Check sheet for the modelled part. Datum: model origin and axes. Units: mm. A direction names the side the tool comes from. Give positions to 0.01 mm unless a question says otherwise; leave off trailing zeros. Order: outer loops, then holes, each group sorted by start corner. A loop starts at its lowest first (then second) coordinate and runs counter-clockwise, first axis right, second up.
from build123d import *

# Parameters (mm, degrees)
F0_R     = 13.786
F0_R_2   = 11.5
F1_DEPTH = 107.95
F2_R     = 13.786
F2_R_2   = 11.5
F3_DEPTH = 31.75
F3_TAPER = 50
F4_T     = 2.54
F5_COUNT = 4
F6_R     = 2.54
F6_2_R   = 2.54
F6_3_R   = 2.54
F6_4_R   = 2.54


# Not quite as in the source:
# - a shell that OpenCascade refuses in one call is made with other operations: the cavity is built on its own and cut out
# - a feature names something its author has since deleted; it is built from what else it names


with BuildPart() as f1:
    # F0 (on Top) → F1 (new body)
    with BuildSketch(Plane.XY):
        Circle(F0_R)
        Circle(F0_R_2, mode=Mode.SUBTRACT)
    extrude(amount=F1_DEPTH)

    # F2 (on face) → F3 (join)
    with BuildSketch(Plane.XY.offset(107.95)):
        Circle(F2_R)
        Circle(F2_R_2, mode=Mode.SUBTRACT)
        Circle(F2_R_2)
    extrude(amount=F3_DEPTH, taper=F3_TAPER)

    # F4: shell of thickness 2.54, made by hand


with BuildPart() as f4_core1:
    # F4_t2: copy of F1
    add(f1.part)

    # the walls: a layer under each face that stays
    f4_faces = [f4_core1.faces().sort_by_distance(p)[0] for p in [
        (-13.786, 0, 53.975),
        (-9.1906666667, -9.1906666667, 0),
        (-6.893, 0, 113.7339137577),
        (-11.5, 0, 53.975),
    ]]
    thicken(f4_faces, amount=-F4_T, mode=Mode.SUBTRACT)


with BuildPart() as f1_1:
    add(f1.part)

    # what is left inside the walls is the cavity
    f4_cavity = [f4_core1.part.solids().sort_by_distance(p)[0] for p in [
        (-6.539981, 0, 110.68124),
    ]]
    add(f4_cavity, mode=Mode.SUBTRACT)


with BuildPart() as f5_1:
    # F5: instance of F1
    add(f1_1.part.rotate(Axis((0, 0, 0), (0, 0, 1)), 1 * 360 / F5_COUNT))

    # F6#2
    f6_2_edges = [f5_1.edges().sort_by_distance(p)[0] for p in [
        (0, -13.786, 107.95),
    ]]
    fillet(f6_2_edges, radius=F6_2_R)


with BuildPart() as f5_2:
    # F5: instance of F1
    add(f1_1.part.rotate(Axis((0, 0, 0), (0, 0, 1)), 2 * 360 / F5_COUNT))

    # F6#3
    f6_3_edges = [f5_2.edges().sort_by_distance(p)[0] for p in [
        (13.786, 0, 107.95),
    ]]
    fillet(f6_3_edges, radius=F6_3_R)


with BuildPart() as f5_3:
    # F5: instance of F1
    add(f1_1.part.rotate(Axis((0, 0, 0), (0, 0, 1)), 3 * 360 / F5_COUNT))

    # F6#4
    f6_4_edges = [f5_3.edges().sort_by_distance(p)[0] for p in [
        (0, 13.786, 107.95),
    ]]
    fillet(f6_4_edges, radius=F6_4_R)


with BuildPart() as f1_2:
    add(f1_1.part)

    # F6
    f6_edges = [f1_2.edges().sort_by_distance(p)[0] for p in [
        (-13.786, 0, 107.95),
        (6.893, 0, 113.733914),
    ]]
    fillet(f6_edges, radius=F6_R)


solid = f1_2.part
1) Set-up check for faces 4 (the face through (-1.5, 11.4, 53.2)), 5 (the face through (-1.632, -1.251, 117.792)): record each of +Z, -Z, +X, -X, +Y, -Y from which the full face is reachable in a straight line by a thin tool's end or side.
Recorded:
face 4: -Z
face 5: +Z
2) Draft check along X on faces 1 (the face through (-1.79, 13.67, 52.64)), 2 (the face through (-0.34, -1.533, 114.885)), 3 (the face through (-9.3, -7.1, 0)). Enter one of: +X half, -X half, draft (parallel to the pull), parting line (faces both ways), or undercut.
Recorded:
face 1: parting line
face 2: undercut
face 3: draft
3) Material ranges on L1, parallel to Y at x = 0, z = 62.5; L2, parallel to X at y = 6.5, z = 81; L3, parallel to X at y = -3, z = 89.5, recorded low to high.
Recorded:
L1: y = -13.79 to -11.5, 11.5 to 13.79
L2: x = -12.16 to -9.49, 9.49 to 12.16
L3: x = -13.46 to -11.1, 11.1 to 13.46
4) Depth check by flat-ended pin: pin 1 Ø2 at (x, z) = (-5, 74) entering from +Y; pin 2 Ø11.5 at (x, y) = (0, 2.5) entering from -Z; pin 3 Ø1 at (x, y) = (-4, -1) entering from -Z. Enter the tip coordinate at first touch or a pass-through.
Recorded:
pin 1: stops at y = 13.19
pin 2: stops at z = 109.28
pin 3: stops at z = 112.32
5) Section check A-A, the plane z = 98. Record the cut outline in (x, y), then the cut area to 3 significant figures.
Recorded:
outline: circle Ø27.57 at (0, 0); hole circle Ø23 at (0, 0)
area: 182 mm2
